Autodesk Fusion 360 part; units mm, degrees
sketch "Sketch1" plane through (0, 0, 0) normal (0, 1, 0) x (1, 0, 0)
  line L0 (0, 0) -> (15, 0)
  line L1 (15, 0) -> (15, -80)
  line L2 (15, -80) -> (0, -80)
  line L3 (0, -80) -> (0, 0)
  dimension "d4" = 15
  dimension "d5" = 80
extrude "Extrude1" add sketch "Sketch1" along normal blind 5
sketch "Sketch3" plane through (0, 5, 0) normal (0, 1, 0) x (-1, 0, 0)
  line L0 (0, 80) -> (-15, 80)
  line L1 (-15, 80) -> (-15, 0)
  line L2 (-15, 0) -> (0, 0)
  line L3 (0, 0) -> (0, 80)
  line L4 (-15, 0) -> (-10, 0)
  line L5 (-10, 0) -> (-10, 8)
  line L6 (-10, 8) -> (-15, 8)
  line L7 (-15, 8) -> (-15, 0)
  dimension "d10" = 5
  dimension "d11" = 8
extrude "Extrude2" add sketch "Sketch3" along normal blind 35 contours L1 L2 L4 L5 L6 L7
sketch "Sketch4" plane through (15, 0, 0) normal (1, 0, 0) x (0, 1, 0)
  line L0 (0, 80) -> (0, 0)
  line L1 (0, 0) -> (40, 0)
  line L2 (40, 0) -> (40, 8)
  line L3 (40, 8) -> (5, 8)
  line L4 (5, 8) -> (5, 80)
  line L5 (5, 80) -> (0, 80)
  line L6 (5, 80) -> (40, 8)
  line L7 (40, 8) -> (5, 8)
  line L8 (5, 8) -> (5, 80)
extrude "Extrude4" add 1 faces at (10, 1.6667, 80) along direction (0, 0, 1) blind 2
extrude "Extrude6" cut 1 faces at (13.3333, 40, 5.3333) along direction (0, -1, 0) blind 8
sketch "Sketch6" plane through (15, 0, 0) normal (1, 0, 0) x (0, 1, 0)
  line L0 (32, 0) -> (32, 8)
  line L1 (32, 8) -> (5, 8)
  line L2 (5, 8) -> (5, 82)
  line L3 (5, 82) -> (0, 82)
  line L4 (0, 82) -> (0, 0)
  line L5 (0, 0) -> (32, 0)
  line L6 (5, 82) -> (5, 8)
  line L7 (5, 8) -> (32, 8)
  line L8 (32, 8) -> (5, 82)
extrude "Extrude7" add sketch "Sketch6" against normal blind 5 contours L1 L2 L6 L7 L8
sketch "Sketch7" plane through (0, 0, 0) normal (0, 0, -1) x (1, 0, 0)
  line L0 (10, -32) -> (15, -32)
  line L1 (15, -32) -> (15, 0)
  line L2 (15, 0) -> (0, 0)
  line L3 (0, 0) -> (0, -5)
  line L4 (0, -5) -> (10, -5)
  line L5 (10, -5) -> (10, -32)
  line L6 (10, -32) -> (10, -5)
  line L7 (10, -5) -> (0, -5)
  line L8 (0, -5) -> (10, -32)
extrude "Extrude8" add sketch "Sketch7" against normal blind 3 contours L4 L5 L6 L7 L8
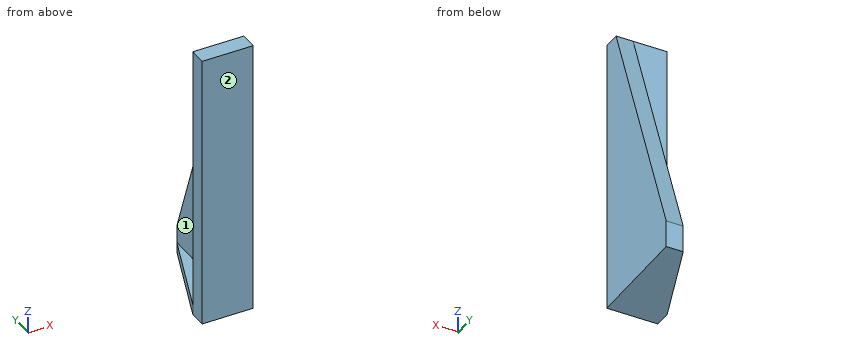
The model under review builds one solid part; all positions refer to its coordinate system, in mm. Face numbers are marked on the shaded views. A direction names the side the tool comes from. Coordinates: 2 decimals unless noted, no trailing zeros. Write each loop counter-clockwise with the first axis right and the second up, starting at its lowest first coordinate (ties: lowest second). Pieces come first, ordered by that corner, then holes. Notation, with made-up numbers: M 83.25,88 L 114.25,88 A15 cw 114.25,101 Z; hole C -11.5,38 d7. An arc over 180 degrees is marked long. Put each result on its own line as item: value.
1) Add section B-B on z = 32. Give the boundary of the cut face in (x, y).
Computed:
outline: M 0,0 L 15,0 L 15,23.24 L 10,23.24 L 10,5 L 0,5 Z
2) Add section A-A on x = 3.5. Give the boundary of the cut face in (y, z).
Computed:
outline: M 0,0 L 14.45,0 L 14.45,3 L 5,3 L 5,82 L 0,82 Z
3) Wall thickness on probe 1 along Y at (x, z) = (8.25, 72); probe 2 along X at (y, z) = (12.5, 49.5); probe 3 along Z at (x, y) = (4, 7): over which ranges is each line inside the solid? List them lowest first. Write a range as [from, to].
Computed:
probe 1: y = [0, 5]
probe 2: x = [10, 15]
probe 3: z = [0, 3]
4) For the marked faces 1 and 2, list the 3-axis set-ups (+Z, -Z, +X, -X, +Y, -Y) from which the entire face can be reached by the end or side of a thin tool; tool diameter is ignored.
Computed:
face 1: +Z, -X, +Y
face 2: +Z, -Z, +X, -X, -Y
5) Clearance check with flat-ended pins moving along their axes: pin 1 Ø5 at (x, y) = (3.5, 25) entering from +Z; pin 2 Ø3 at (x, z) = (7, 29) entering from +Y; pin 3 Ø8 at (y, z) = (17.5, 37) entering from -X. State where each tip first meets the part, or that it passes through.
Computed:
pin 1: passes through
pin 2: stops at y = 5
pin 3: stops at x = 10
